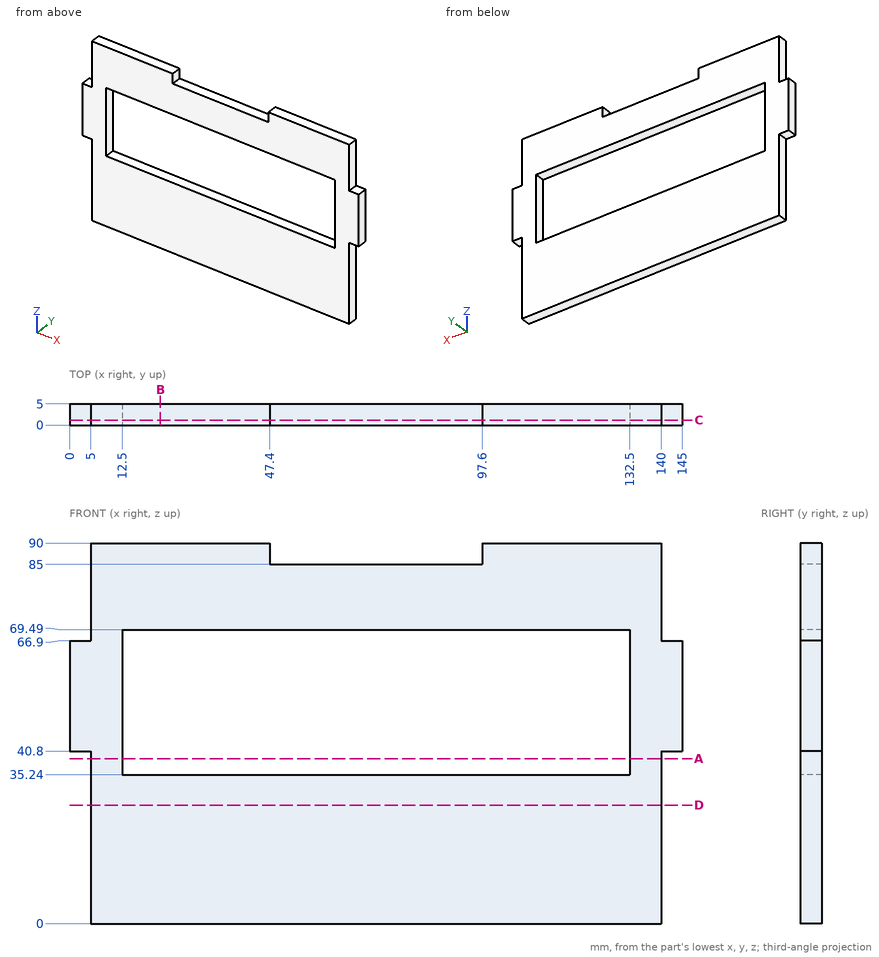
Input: dimensioned drawing with shaded views. Units: mm. Origin: part minimum x, y, z. Round coordinates to 2 decimals unless told otherwise and drop trailing zeros. Loops run counter-clockwise (first coordinate to the right, second up) from the corner with the lowest first, then second, coordinate; pieces in that order, holes last. Notation, with made-up numbers: M 25.25,20.5 L 67.25,20.5 A31 cw 67.25,52.5 Z; hole C -21,84 d5. An arc over 180 degrees is marked long. Return JSON: item names as keys, results as strings. Group by question number.
1. Section query B-B on x = 21.5. Output: boundary loops of the cut face in (y, z).
2. Pin query (flat end, axial travel): pin 1 (1.5 mm diameter, centred on x = 142.5, y = 3.5, fed in from +Z); pin 2 (1.5 mm diameter, centred on y = 3, z = 77.5, fed in from -X); pin 3 (1.5 mm diameter, centred on y = 2.5, z = 23, fed in from +X). Return the tip coordinate at first contact, or that it passes through.
3. Section query C-C on y = 1.2. Output: boundary loops of the cut face in (x, z), and give its area (3 significant figures).
4. Section query D-D on z = 28. Output: boundary loops of the cut face in (x, y), and give its area (3 significant figures).
5. Section query A-A on z = 39. Output: boundary loops of the cut face in (x, y).
6. Material intervals for line 1 along Z through (x, y) = (114.5, 4.4); line 2 along X through (y, z) = (1.35, 61); line 3 along Z through (x, y) = (78, 0.3), sorted ascending. Write a range as from..to.
Checks:
{
 "1": {"outline": "M 0,0 L 5,0 L 5,35.24 L 0,35.24 Z; M 0,69.49 L 5,69.49 L 5,90 L 0,90 Z"},
 "2": {"pin 1": "stops at z = 66.9", "pin 2": "stops at x = 5", "pin 3": "stops at x = 140"},
 "3": {"outline": "M 0,40.8 L 5,40.8 L 5,0 L 140,0 L 140,40.8 L 145,40.8 L 145,66.9 L 140,66.9 L 140,90 L 97.6,90 L 97.6,85 L 47.4,85 L 47.4,90 L 5,90 L 5,66.9 L 0,66.9 Z; hole M 12.5,35.24 L 132.5,35.24 L 132.5,69.49 L 12.5,69.49 Z", "area": "8,050 mm²"},
 "4": {"outline": "M 5,0 L 140,0 L 140,5 L 5,5 Z", "area": "675 mm²"},
 "5": {"outline": "M 5,0 L 12.5,0 L 12.5,5 L 5,5 Z; M 132.5,0 L 140,0 L 140,5 L 132.5,5 Z"},
 "6": {"line 1": "z = 0..35.24, 69.49..90", "line 2": "x = 0..12.5, 132.5..145", "line 3": "z = 0..35.24, 69.49..85"}
}
